CAD build for the part. Positions are in the model's coordinates, mm. Face numbers are marked on the shaded views. Round coordinates to 2 decimals unless told otherwise and drop trailing zeros. Loops run counter-clockwise (first coordinate to the right, second up) from the corner with the lowest first, then second, coordinate; pieces in that order, holes last.
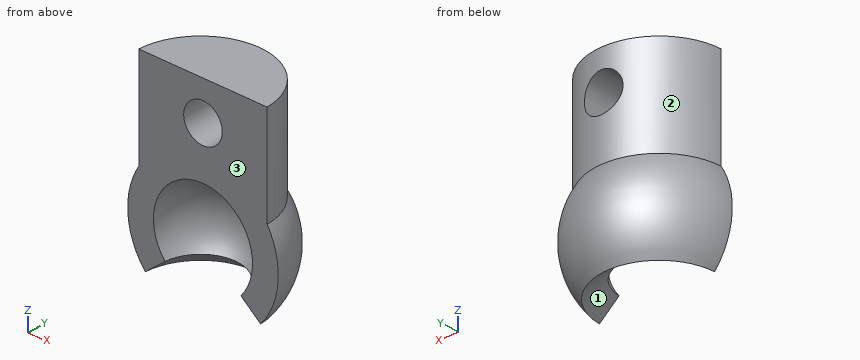
from build123d import *

# Parameters (mm, degrees)
F1_ANGLE = 180
F3_R     = 1.905
F4_DEPTH = 7.4432
F6_DEPTH = 18.576954


with BuildPart() as f1:
    # F0 (on Front) → F1 (revolve)
    with BuildSketch(Plane.XZ):
        with BuildLine():
            ThreePointArc((0, 4.9022), (4.442902, 2.071759), (3.755303, -3.151073))
            Line((3.755303, -3.151073), (5.701056, -4.783754))
            ThreePointArc((5.701056, -4.783754), (7.421416, -0.555811), (6.35, 3.881216))
            Line((6.35, 3.881216), (6.35, 7.3025))
            Line((6.35, 7.3025), (6.35, 13.7922))
            Line((6.35, 13.7922), (0, 13.7922))
            Line((0, 13.7922), (0, 7.4422))
            Line((0, 7.4422), (0, 4.9022))
        make_face()
    revolve(axis=Axis((0, 0, 10.6172), (0, 0, 1)), revolution_arc=F1_ANGLE)

    # F3 (on face) → F4 (cut, through all)
    with BuildSketch(Plane.XZ):
        with Locations((0, 9.9822)):
            Circle(F3_R)
    extrude(amount=-F4_DEPTH, mode=Mode.SUBTRACT)

    # F5 (on face) → F6 (cut, through all)
    with BuildSketch(Plane.XY.offset(13.7922)):
        with BuildLine():
            ThreePointArc((-6.344918, 0.254), (-6.348729, 0.127025), (-6.35, 0))
            Line((-6.35, 0), (6.35, 0))
            ThreePointArc((6.35, 0), (6.348729, 0.127025), (6.344918, 0.254))
            Line((6.344918, 0.254), (-6.344918, 0.254))
        make_face()
        with BuildLine():
            Line((-9.525, 0.254), (-9.525, 0))
            Line((-9.525, 0), (-6.35, 0))
            ThreePointArc((-6.35, 0), (-6.348729, 0.127025), (-6.344918, 0.254))
            Line((-6.344918, 0.254), (-9.525, 0.254))
        make_face()
        with BuildLine():
            ThreePointArc((6.344918, 0.254), (6.348729, 0.127025), (6.35, 0))
            Line((6.35, 0), (9.525, 0))
            Line((9.525, 0), (9.525, 0.254))
            Line((9.525, 0.254), (6.344918, 0.254))
        make_face()
    extrude(amount=-F6_DEPTH, mode=Mode.SUBTRACT)


solid = f1.part
Item 1: Cut at A-A (z = 8.5). List the corners of the cut face in (x, y).
Verdict:
outline: (-6.34, 0.25) - (-1.2, 0.25) - (-1.2, 6.24) arc R6.35 ccw to start; (1.2, 0.25) - (6.34, 0.25) arc R6.35 ccw to (1.2, 6.24) - close
Item 2: Flat gauge pins, fed straight in: P1, Ø1, axis at x = -4, y = 5, coming from the -Z side; P2, Ø2, axis at x = 2.5, z = 0.5, coming from the -Y side; P3, Ø3, axis at y = 6, z = 11.5, coming from the -X side. Where does each tip first touch, or does it go through?
Verdict:
P1: stops at z = -4.53
P2: stops at y = 3.38
P3: stops at x = -4.48
Item 3: Cut at C-C (y = 4.25). State how many separate pieces and enclosed holes the cut face has, plus the area to 3 significant figures.
Verdict:
separate pieces: 1
enclosed holes: 2
area: 153 mm2
Item 4: Wall check: L1, parallel to Z at x = 0, y = 4.25; L2, parallel to Z at x = 0.25, y = 4.5; L3, parallel to Z at x = 0.75, y = 2.5. Give the ranges that are in metal, low to high.
Verdict:
L1: z = -3.57 to -2.44, 2.44 to 8.08, 11.89 to 13.79
L2: z = -3.78 to -1.93, 1.93 to 8.09, 11.87 to 13.79
L3: z = 4.15 to 8.23, 11.73 to 13.79
Item 5: Mould opens along X. For the marked faces 1, 2 and 3 say: released by +X, released by -X, zero draft, split by the parting line, or undercut.
Verdict:
face 1: undercut
face 2: split by the parting line
face 3: zero draft
